```python
from build123d import *

# Parameters (mm, degrees)
BOSS_EXTRUDE1_DEPTH = 3.5
SKETCH2_R           = 1.025
CUT_EXTRUDE1_DEPTH  = 16.321553446


with BuildPart() as part:
    # Sketch1 → Boss-Extrude1 (new body)
    with BuildSketch(Plane.XY):
        with BuildLine():
            Line((-2.491304321, 12.208333333), (-3.48782605, 0.291666667))
            ThreePointArc((-3.48782605, 0.291666667), (0, -3.5), (3.48782605, 0.291666667))
            Line((3.48782605, 0.291666667), (2.491304321, 12.208333333))
            ThreePointArc((2.491304321, 12.208333333), (0, 14.5), (-2.491304321, 12.208333333))
        make_face()
    extrude(amount=BOSS_EXTRUDE1_DEPTH)

    # Sketch2 → Cut-Extrude1 (cut, through all)
    with BuildSketch(Plane.XY.offset(3.5)):
        with Locations((0, 12)):
            Circle(SKETCH2_R)
        with BuildLine():
            Line((-1.118033989, 1), (1.118033989, 1))
            ThreePointArc((1.118033989, 1), (0, -1.5), (-1.118033989, 1))
        make_face()
    extrude(amount=-CUT_EXTRUDE1_DEPTH, mode=Mode.SUBTRACT)


solid = part.part
```
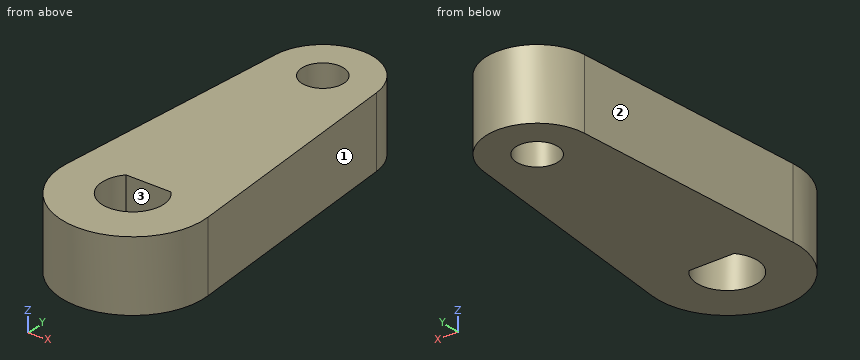
Model file for the job. Use its own axes, mm. Face numbers are marked on the shaded views. Give positions to 0.01 mm unless a question says otherwise; leave off trailing zeros. Write each loop counter-clockwise with the first axis right and the second up, starting at its lowest first coordinate (ties: lowest second). Pieces come first, ordered by that corner, then holes. Notation, with made-up numbers: (-34.75, -16) -> (-11.75, -16) arc R5 cw to (-11.75, -7) -> close; hole circle Ø1 at (-17, 40). An arc over 180 degrees is marked (long way). Use CSV: the item, a comma, the result in double quotes. Start each with the question number.
1) Drill centre lines: L1, parallel to X at y = 0, z = 1.1; L2, parallel to Y at x = 0.5, z = 0.75; L3, parallel to Y at x = -0.25, z = 1.6. Where is each one in solid material? Low to high.
2) Cut at A-A on x = 0. List the corners of the cut face in (y, z) (3 decimals), plus the area to 3 significant figures.
3) Two-plate mould, pull along X, no slides. Class the marked faces 1, 2 and 3: released by +X, released by -X, zero draft, split by the parting line, or undercut.
4) Pin check, flat tip, straight feed: P1, Ø1.5, axis at y = 3.5, z = 0.5, coming from the +X side. Stop position of the tip, or through.
5) Cut at B-B on y = 0. List the corners of the cut face in (x, z).
6) Cut at D-D on y = 13.5. List the corners of the cut face in (x, z).
7) Cut at C-C on z = 2.9. List the corners of the cut face in (x, y) (3 decimals), plus the area to 3 significant figures.
Final values:
1,L1,"x = -3.5 to -1.5, 1.5 to 3.5"
1,L2,"y = -3.46 to -1.41, 1 to 11.11, 12.89 to 14.45"
1,L3,"y = -3.49 to -1.48, 1 to 11.01, 12.99 to 14.49"
2,outline,"(-3.5, 0) -> (-1.5, 0) -> (-1.5, 3.5) -> (-3.5, 3.5) -> close; (1, 0) -> (10.975, 0) -> (10.975, 3.5) -> (1, 3.5) -> close; (13.025, 0) -> (14.5, 0) -> (14.5, 3.5) -> (13.025, 3.5) -> close"
2,area,"47.1 mm2"
3,face 1,"released by +X"
3,face 2,"released by -X"
3,face 3,"undercut"
4,P1,"stops at x = 3.28"
5,outline,"(-3.5, 0) -> (-1.5, 0) -> (-1.5, 3.5) -> (-3.5, 3.5) -> close; (1.5, 0) -> (3.5, 0) -> (3.5, 3.5) -> (1.5, 3.5) -> close"
6,outline,"(-2, 0) -> (2, 0) -> (2, 3.5) -> (-2, 3.5) -> close"
7,outline,"(-3.488, 0.292) arc R3.5 ccw (long way) to (3.488, 0.292) -> (2.491, 12.208) arc R2.5 ccw to (-2.491, 12.208) -> close; hole (-1.118, 1) arc R1.5 ccw (long way) to (1.118, 1) -> close; hole circle Ø2.05 at (0, 12)"
7,area,"91.7 mm2"
